from build123d import *

# Parameters (mm, degrees)
SKETCH1_R           = 1.5
SKETCH1_R_2         = 11.5
BOSS_EXTRUDE1_DEPTH = 5
BOSS_EXTRUDE2_START = -5
SKETCH2_R           = 11.5
SKETCH2_R_2         = 2.7
BOSS_EXTRUDE2_DEPTH = 5
SKETCH3_R           = 1
BOSS_EXTRUDE3_DEPTH = 5
FILLET1_R           = 3


with BuildPart() as part:
    # Sketch1 → Boss-Extrude1 (new body)
    with BuildSketch(Plane.XY):
        Polygon((0, 80), (-80, 80), (-80, 70), (-85, 70), (-85, 65), (-80, 65), (-80, 61.5), (-77, 61.5), (-77, 62.6), (-74.7, 62.6), (-74.7, 61.5), (-70, 61.5), (-70, 58.5), (-74.7, 58.5), (-74.7, 57.4), (-77, 57.4), (-77, 58.5), (-80, 58.5), (-80, 55), (-85, 55), (-85, 50), (-80, 50), (-80, 30), (-85, 30), (-85, 25), (-80, 25), (-80, 21.5), (-77, 21.5), (-77, 22.6), (-74.7, 22.6), (-74.7, 21.5), (-70, 21.5), (-70, 18.5), (-74.7, 18.5), (-74.7, 17.4), (-77, 17.4), (-77, 18.5), (-80, 18.5), (-80, 15), (-85, 15), (-85, 10), (-80, 10), (-80, 0), (0, 0), (0, 10), (5, 10), (5, 15), (0, 15), (0, 18.5), (-3, 18.5), (-3, 17.4), (-5.3, 17.4), (-5.3, 18.5), (-10, 18.5), (-10, 21.5), (-5.3, 21.5), (-5.3, 22.6), (-3, 22.6), (-3, 21.5), (0, 21.5), (0, 25), (5, 25), (5, 30), (0, 30), (0, 50), (5, 50), (5, 55), (0, 55), (0, 58.5), (-3, 58.5), (-3, 57.4), (-5.3, 57.4), (-5.3, 58.5), (-10, 58.5), (-10, 61.5), (-5.3, 61.5), (-5.3, 62.6), (-3, 62.6), (-3, 61.5), (0, 61.5), (0, 65), (5, 65), (5, 70), (0, 70), align=None)
        with Locations((-55.922, 70.922)):
            Circle(SKETCH1_R, mode=Mode.SUBTRACT)
        with Locations((-24.078, 70.922)):
            Circle(SKETCH1_R, mode=Mode.SUBTRACT)
        with Locations((-24.078, 39.078)):
            Circle(SKETCH1_R, mode=Mode.SUBTRACT)
        with Locations((-55.922, 39.078)):
            Circle(SKETCH1_R, mode=Mode.SUBTRACT)
        with Locations((-40, 55)):
            Circle(SKETCH1_R_2, mode=Mode.SUBTRACT)
    extrude(amount=BOSS_EXTRUDE1_DEPTH)

    # Sketch2 → Boss-Extrude2 (add)
    with BuildSketch(Plane.XY.offset(5).offset(BOSS_EXTRUDE2_START)):
        with Locations((-40, 55)):
            Circle(SKETCH2_R)
        with Locations((-40, 55)):
            Circle(SKETCH2_R_2, mode=Mode.SUBTRACT)
    extrude(amount=BOSS_EXTRUDE2_DEPTH)

    # Sketch3 → Boss-Extrude3 (add)
    with BuildSketch(Plane.XY.offset(5)):
        Polygon((5, 125), (-14.5, 125), (-37, 80), (-10, 80), (-10, 90), (5, 120), align=None)
        with Locations((-9.5, 120)):
            Circle(SKETCH3_R, mode=Mode.SUBTRACT)
        with Locations((0, 120)):
            Circle(SKETCH3_R, mode=Mode.SUBTRACT)
    extrude(amount=-BOSS_EXTRUDE3_DEPTH)

    # Fillet1
    fillet1_edges = [part.edges().sort_by_distance(p)[0] for p in [
        (-10, 90, 2.5),
        (-10, 80, 2.5),
        (-37, 80, 2.5),
        (-14.5, 125, 2.5),
        (5, 125, 2.5),
        (5, 120, 2.5),
    ]]
    fillet(fillet1_edges, radius=FILLET1_R)


solid = part.part
Could you check a few things on this model? Use its own coordinates, in mm. A direction names the side the tool comes from. Give positions to 0.01 mm unless a question says otherwise; leave off trailing zeros. Loops run counter-clockwise (first coordinate to the right, second up) from the corner with the lowest first, then second, coordinate; pieces in that order, holes last. Notation, with made-up numbers: (27, 38.25) -> (53, 38.25) arc R16 ccw to (53, 44.25) -> close; hole circle Ø10 at (36, 1). An arc over 180 degrees is marked (long way). Return JSON: item names as keys, results as strings.
Item 1: I need wall thicknesses on L1, parallel to X at y = 22.5, z = 3.4; L2, parallel to Y at x = -9.5, z = 3; L3, parallel to Y at x = -5.5, z = 3.3. Which ranges of each line are inside material? Lowest first, please. Write a range as from..to.
Geometry results:
{"L1": "x = -80..-77, -74.7..-5.3, -3..0", "L2": "y = 0..18.5, 21.5..58.5, 61.5..81.34, 91..119, 121..125", "L3": "y = 0..18.5, 21.5..58.5, 61.5..80, 99..125"}
Item 2: If we section it at C-C on z = 1.1: Count the separate pieces of the cut face and the enclosed holes in it, plus the area to 3 significant figures.
Geometry results:
{"separate pieces": "1", "enclosed holes": "7", "area": "7,410 mm²"}
Item 3: If we section it at A-A on x = -53: List the corners of the cut face in (y, z) for me.
Geometry results:
{"outline": "(0, 0) -> (80, 0) -> (80, 5) -> (0, 5) -> close"}
Item 4: We'd pull the mould along Y, two halves only. Please class faces 1 (the flat face through (5, 67, 2)), 2 (the cylindrical face through (-37.297, 80.436, 2.465)), 3 (the flat face through (0, 23, 2)): +Y half, -Y half, draft (parallel to the pull), parting line (faces both ways), or undercut.
Geometry results:
{"face 1": "draft", "face 2": "+Y half", "face 3": "undercut"}
Item 5: I'm going to push flat-ended pins straight in: pin 1 (1.5 mm diameter, centred on x = -78, z = 1.5, fed in from +Y); pin 2 (1.5 mm diameter, centred on x = 2, z = 1.5, fed in from -Y); pin 3 (1 mm diameter, centred on y = 39, z = 2.5, fed in from -X); pin 4 (5 mm diameter, centred on x = -30.5, y = 103, fed in from -Z). Where does each tip first touch, or does it pass through?
Geometry results:
{"pin 1": "stops at y = 80", "pin 2": "stops at y = 10", "pin 3": "stops at x = -80", "pin 4": "passes through"}
Item 6: Which directions (+Z, -Z, +X, -X, +Y, -Y) give clear straight access to the entire face, cutting with the end or side of a thin tool? Please do faces 4 (the flat face through (-82, 15, 2)), 5 (the flat face through (-59, 80, 2)), 6 (the flat face through (-1, 18.5, 2)).
Geometry results:
{"face 4": "+Z, -Z, -X", "face 5": "+Z, -Z, -X, +Y", "face 6": "+Z, -Z, +X"}
Item 7: If we section it at B-B on y = 114: List the corners of the cut face in (x, z) for me, plus the area to 3 significant figures.
Geometry results:
{"outline": "(-20, 0) -> (2, 0) -> (2, 5) -> (-20, 5) -> close", "area": "110 mm²"}
